Check sheet for the drawn part. Datum: minimum x, y, z corner. Units: mm. A direction names the side the tool comes from. Give positions to 0.01 mm unless a question says otherwise; leave off trailing zeros. Loops run counter-clockwise (first coordinate to the right, second up) from the corner with the lowest first, then second, coordinate; pieces in that order, holes last.
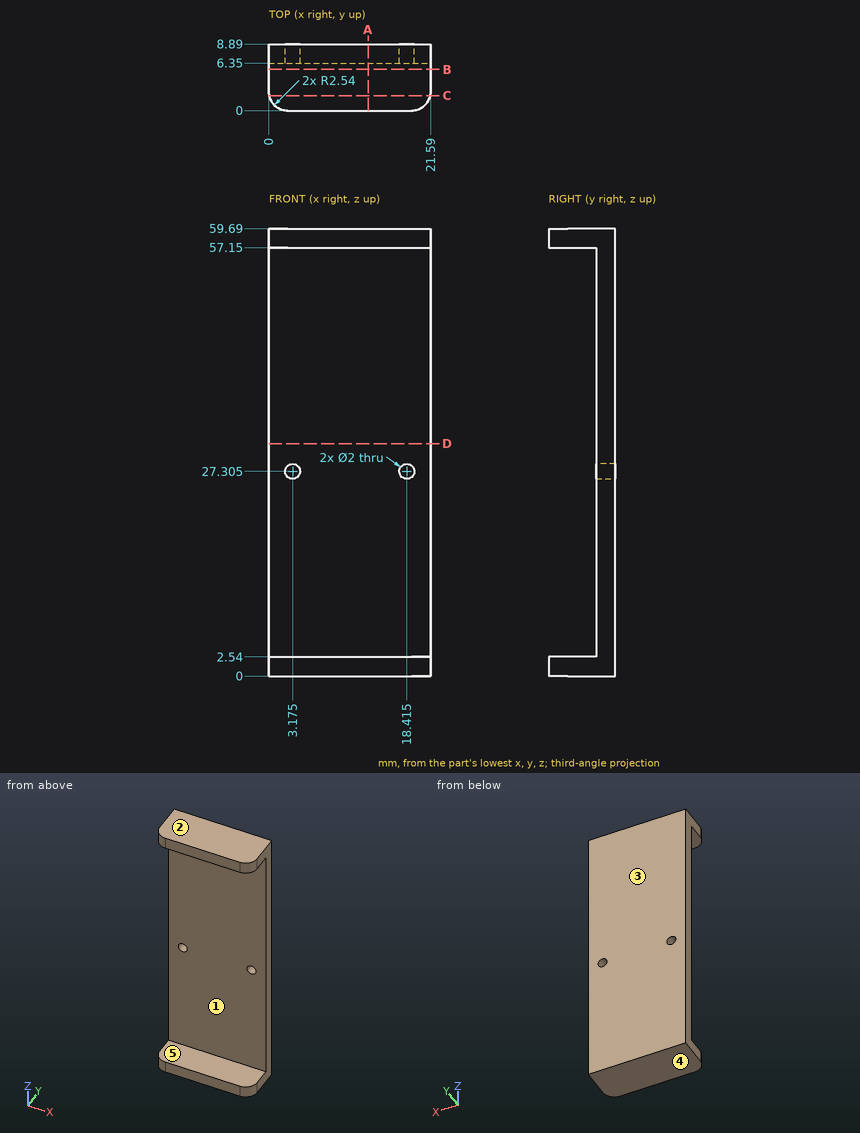
(1) Section check B-B on y = 5.5. Record the boundary of the cut face in (x, z).
(2) Release check for a two-part mould opening along Z. For the marked faces 1, 2 and 3 record: pulls with the +Z half, pulls with the -Z half, needs draft (parallel to the pull), parting line crosses it, or undercut.
(3) Section check D-D on z = 31. Record the boundary of the cut face in (x, y).
(4) Section check A-A on x = 13.25. Record the boundary of the cut face in (y, z).
(5) Gauge pin test, flat ends, axial feed: pin 1 Ø2 at (x, z) = (19, 38) entering from -Y; pin 2 Ø1.6 at (x, z) = (3.175, 27.305) entering from +Y (1 decimal). Record the tip position at first contact, or that the pin passes through.
(6) Access from +Z, -Z, +X, -X, +Y, -Y to the whole of each face (thin tool, end or side, straight path). Record for the marked faces 4 and 5.
(7) Material ranges on line 1 (Z direction, x = 18.75, y = 0.75); line 2 (X direction, y = 7, z = 26.5); line 3 (Y direction, x = 18, z = 40.5), recorded low to high.
(8) Section check C-C on y = 2. Record the boundary of the cut face in (x, z).
Computed values:
1. outline: (0, 0) - (21.59, 0) - (21.59, 2.54) - (0, 2.54) - close; (0, 57.15) - (21.59, 57.15) - (21.59, 59.69) - (0, 59.69) - close
2. face 1: undercut
2. face 2: pulls with the +Z half
2. face 3: needs draft
3. outline: (0, 6.35) - (21.59, 6.35) - (21.59, 8.89) - (0, 8.89) - close
4. outline: (0, 0) - (8.89, 0) - (8.89, 59.69) - (0, 59.69) - (0, 57.15) - (6.35, 57.15) - (6.35, 2.54) - (0, 2.54) - close
5. pin 1: stops at y = 6.35
5. pin 2: passes through
6. face 4: -Z, +X, -X, +Y, -Y
6. face 5: +X, -X, -Y
7. line 1: z = 0 to 2.54, 57.15 to 59.69
7. line 2: x = 0 to 2.58, 3.77 to 17.82, 19.01 to 21.59
7. line 3: y = 6.35 to 8.89
8. outline: (0.06, 0) - (21.53, 0) - (21.53, 2.54) - (0.06, 2.54) - close; (0.06, 57.15) - (21.53, 57.15) - (21.53, 59.69) - (0.06, 59.69) - close
